CAD build for the part. Positions are in the model's coordinates, mm. Give positions to 0.01 mm unless a question says otherwise; leave off trailing zeros. Write each loop counter-clockwise with the first axis right and the second up, starting at its lowest first coordinate (ties: lowest second). Pieces come first, ordered by that corner, then holes. Notation, with made-up numbers: (-18, 62.5) - (17, 62.5) arc R25 ccw to (17, 99.5) - close; hole circle Ø9 at (45.5, -18.75). An arc over 180 degrees is marked (long way). Put each result on its own line as item: value. Start each with the question number.
1. Wall check: line 1 (X direction, y = 6.5, z = 0); line 2 (X direction, y = 0.5, z = 2); line 3 (Z direction, x = -6.5, y = 4.25). Give the ranges that are in metal, low to high.
2. Mould opens along Z. For faces 1 (the flat face through (0, 10, 0)), 2 (the cylindrical face through (-1.63, 4.93, 0.44)), 3 (the flat face through (0, 5, 15)) say: +Z half, -Z half, draft (parallel to the pull), parting line (faces both ways), or undercut.
3. Cut at A-A on x = -20. List the corners of the cut face in (y, z).
4. Drop a flat-ended pin along its axis: pin 1 (4 mm diameter, centred on x = -20, z = 0, fed in from +Y). Give the stop position or say it passes through.
5. Cut at B-B on z = 0. List the corners of the cut face in (x, y), and give its area (3 significant figures).
6. Cut at D-D on x = 20. List the corners of the cut face in (y, z).
7. Cut at C-C on y = 4.25. List the corners of the cut face in (x, z).
from build123d import *

# Parameters (mm, degrees)
SKETCH_1_W         = 60
SKETCH_1_H         = 30
EXTRUDE_1_DEPTH    = 10
MM_1_D             = 6.8
HOLE_WIZARD_M6_1_D = 5


with BuildPart() as part:
    # 草图1 → 凸台-拉伸1 (new body)
    with BuildSketch(Plane(origin=(0, 0, 0), x_dir=(1, 0, 0), z_dir=(0, 1, 0))):
        Rectangle(SKETCH_1_W, SKETCH_1_H)
    extrude(amount=EXTRUDE_1_DEPTH)

    # 大小mm 暗销孔1 (through all)
    with Locations(Plane(origin=(-20, 10, 0), x_dir=(0, 0, 1), z_dir=(0, 1, 0))):
        with Locations((0, 0), (0, 15)):
            Hole(MM_1_D / 2)

    # M6 螺纹孔1 (through all)
    with Locations(Plane(origin=(20, 10, 0), x_dir=(0, 0, 1), z_dir=(0, 1, 0))):
        with Locations((0, 0)):
            Hole(HOLE_WIZARD_M6_1_D / 2)


solid = part.part
Report:
1. line 1: x = -30 to -23.4, -16.6 to -8.4, -1.6 to 17.5, 22.5 to 30
1. line 2: x = -30 to -22.75, -17.25 to -7.75, -2.25 to 18.5, 21.5 to 30
1. line 3: z = -15 to -3.05, 3.05 to 15
2. face 1: draft
2. face 2: undercut
2. face 3: +Z half
3. outline: (0, -15) - (10, -15) - (10, -3.4) - (0, -3.4) - close; (0, 3.4) - (10, 3.4) - (10, 15) - (0, 15) - close
4. pin 1: passes through
5. outline: (-30, 0) - (-23.4, 0) - (-23.4, 10) - (-30, 10) - close; (-16.6, 0) - (-8.4, 0) - (-8.4, 10) - (-16.6, 10) - close; (-1.6, 0) - (17.5, 0) - (17.5, 10) - (-1.6, 10) - close; (22.5, 0) - (30, 0) - (30, 10) - (22.5, 10) - close
5. area: 414 mm²
6. outline: (0, -15) - (10, -15) - (10, -2.5) - (0, -2.5) - close; (0, 2.5) - (10, 2.5) - (10, 15) - (0, 15) - close
7. outline: (-30, -15) - (30, -15) - (30, 15) - (-30, 15) - close; hole circle Ø6.8 at (-20, 0); hole circle Ø6.8 at (-5, 0); hole circle Ø5 at (20, 0)
